Here's how the part is built. I have some questions about the finished solid (model axes, mm). Face numbers are marked on the shaded views. A direction names the side the tool comes from. Coordinates: 2 decimals unless noted, no trailing zeros. Write each loop counter-clockwise with the first axis right and the second up, starting at its lowest first coordinate (ties: lowest second). Pieces come first, ordered by that corner, then holes. Notation, with made-up numbers: (55.25, 88) -> (72.25, 88) arc R13 cw to (72.25, 108) -> close; hole circle Ø9 at (-19.5, -17). An arc over 180 degrees is marked (long way). Put each result on its own line as item: value.
```python
from build123d import *

# Parameters (mm, degrees)
BOSS_EXTRUDE1_DEPTH                             = 42
CUT_EXTRUDE1_DEPTH                              = 3
CUT_EXTRUDE2_DEPTH                              = 2
CSK_FOR_M3_FLAT_HEAD_MACHINE_SCREW1_D           = 3.4
CSK_FOR_M3_FLAT_HEAD_MACHINE_SCREW1_CSINK_D     = 6.3
CSK_FOR_M3_FLAT_HEAD_MACHINE_SCREW1_CSINK_ANGLE = 90
FILLET3_R                                       = 1
FILLET4_R                                       = 1
FILLET5_R                                       = 1
FILLET6_R                                       = 1
FILLET7_R                                       = 1
FILLET8_R                                       = 1


with BuildPart() as part:
    # Sketch1 → Boss-Extrude1 (new body)
    with BuildSketch(Plane.XY):
        Polygon((-124.373548005, 69.489611766), (-124.373548005, 24.489611766), (-109.373548005, 24.489611766), (-109.373548005, 28.489611766), (-120.373548005, 28.489611766), (-120.373548005, 69.489611766), align=None)
    extrude(amount=BOSS_EXTRUDE1_DEPTH)

    # Sketch2 → Cut-Extrude1 (cut)
    with BuildSketch(Plane(origin=(-120.373548005, 0, 0), x_dir=(0, 0, -1), z_dir=(1, 0, 0))):
        with BuildLine():
            Line((-42, 52.639611766), (-30, 52.639611766))
            ThreePointArc((-30, 52.639611766), (-26.35, 48.989611766), (-30, 45.339611766))
            Line((-30, 45.339611766), (-42, 45.339611766))
            Line((-42, 45.339611766), (-42, 52.639611766))
        make_face()
    cut_extrude1 = extrude(amount=-CUT_EXTRUDE1_DEPTH, mode=Mode.SUBTRACT)

    # Sketch4 → Cut-Extrude2 (cut, through all)
    with BuildSketch(Plane(origin=(-123.373548005, 0, 0), x_dir=(0, 0, -1), z_dir=(1, 0, 0))):
        with BuildLine():
            Line((-42, 51.189611766), (-42, 46.789611766))
            Line((-42, 46.789611766), (-30, 46.789611766))
            ThreePointArc((-30, 46.789611766), (-27.8, 48.989611766), (-30, 51.189611766))
            Line((-30, 51.189611766), (-42, 51.189611766))
        make_face()
    cut_extrude2 = extrude(amount=-CUT_EXTRUDE2_DEPTH, mode=Mode.SUBTRACT)

    # Mirror2: Cut-Extrude1, Cut-Extrude2 across plane
    add(cut_extrude1.mirror(Plane.XY.offset(21)), mode=Mode.SUBTRACT)
    add(cut_extrude2.mirror(Plane.XY.offset(21)), mode=Mode.SUBTRACT)

    # CSK for M3 Flat Head Machine Screw1 (through all)
    with Locations(Plane(origin=(0, 28.489611766, 0), x_dir=(1, 0, 0), z_dir=(0, 1, 0))):
        with Locations((-114.873548005, -32), (-114.873548005, -10)):
            CounterSinkHole(CSK_FOR_M3_FLAT_HEAD_MACHINE_SCREW1_D / 2, CSK_FOR_M3_FLAT_HEAD_MACHINE_SCREW1_CSINK_D / 2, counter_sink_angle=CSK_FOR_M3_FLAT_HEAD_MACHINE_SCREW1_CSINK_ANGLE)

    # Fillet3
    fillet3_edges = [part.edges().sort_by_distance(p)[0] for p in [
        (-120.373548005, 36.914611766, 42),
    ]]
    fillet(fillet3_edges, radius=FILLET3_R)

    # Fillet4
    fillet4_edges = [part.edges().sort_by_distance(p)[0] for p in [
        (-120.373548005, 61.064611766, 42),
    ]]
    fillet(fillet4_edges, radius=FILLET4_R)

    # Fillet5
    fillet5_edges = [part.edges().sort_by_distance(p)[0] for p in [
        (-120.666441224, 52.639611766, 41.707106781),
        (-122.373548005, 45.339611766, 42),
        (-122.373548005, 52.639611766, 42),
        (-120.373548005, 48.989611766, 26.35),
        (-120.373548005, 52.639611766, 35.5),
        (-120.373548005, 45.339611766, 35.5),
        (-120.666441224, 45.339611766, 41.707106781),
    ]]
    fillet(fillet5_edges, radius=FILLET5_R)

    # Fillet6
    fillet6_edges = [part.edges().sort_by_distance(p)[0] for p in [
        (-122.873548005, 69.489611766, 42),
        (-120.666441224, 69.489611766, 41.707106781),
        (-114.873548005, 28.489611766, 42),
        (-109.373548005, 28.489611766, 21),
        (-114.873548005, 28.489611766, 0),
        (-120.373548005, 36.914611766, 0),
        (-120.373548005, 48.989611766, 15.65),
        (-120.373548005, 45.339611766, 6),
        (-120.373548005, 52.639611766, 6),
        (-120.373548005, 61.064611766, 0),
        (-120.373548005, 69.489611766, 20.5),
    ]]
    fillet(fillet6_edges, radius=FILLET6_R)

    # Fillet7
    fillet7_edges = [part.edges().sort_by_distance(p)[0] for p in [
        (-123.873548005, 51.189611766, 42),
    ]]
    fillet(fillet7_edges, radius=FILLET7_R)

    # Fillet8
    fillet8_edges = [part.edges().sort_by_distance(p)[0] for p in [
        (-123.873548005, 46.789611766, 42),
        (-123.873548005, 51.189611766, 0),
        (-123.873548005, 46.789611766, 0),
    ]]
    fillet(fillet8_edges, radius=FILLET8_R)


solid = part.part
```
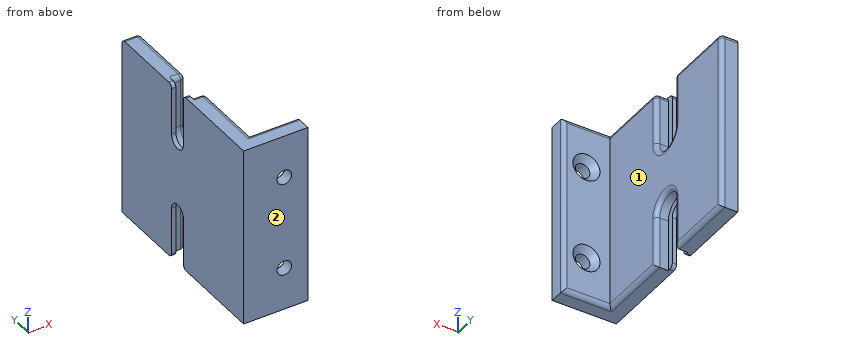
Item 1: Please list where these lines run through material, in increasing order: line 1 along Y through (x, z) = (-121.5, 3.5); line 2 along Y through (x, z) = (-118, 20.5); line 3 along X through (y, z) = (26, 10). Write a range as from..to.
Output:
line 1: y = 24.49..45.34, 52.64..69.49
line 2: y = 24.49..28.49
line 3: x = -124.37..-116.57, -113.17..-109.37
Item 2: Imagine slicing it at C-C on z = 10. Write out the boundary of the cut face in (x, y).
Output:
outline: (-124.37, 24.49) -> (-116.57, 24.49) -> (-116.57, 27.04) -> (-118.02, 28.49) -> (-120.37, 28.49) -> (-120.37, 44.34) arc R1 ccw to (-121.37, 45.34) -> (-123.37, 45.34) -> (-123.37, 46.79) -> (-124.37, 46.79) -> close; (-124.37, 51.19) -> (-123.37, 51.19) -> (-123.37, 52.64) -> (-121.37, 52.64) arc R1 ccw to (-120.37, 53.64) -> (-120.37, 68.49) arc R1 ccw to (-121.37, 69.49) -> (-124.37, 69.49) -> close; (-113.17, 24.49) -> (-109.37, 24.49) -> (-109.37, 27.49) arc R1 ccw to (-110.37, 28.49) -> (-111.72, 28.49) -> (-113.17, 27.04) -> close
Item 3: Imagine slicing it at A-A on z = 4. Write out the boundary of the cut face in (x, y).
Output:
outline: (-124.37, 24.49) -> (-109.37, 24.49) -> (-109.37, 27.49) arc R1 ccw to (-110.37, 28.49) -> (-120.37, 28.49) -> (-120.37, 44.34) arc R1 ccw to (-121.37, 45.34) -> (-123.37, 45.34) -> (-123.37, 46.79) -> (-124.37, 46.79) -> close; (-124.37, 51.19) -> (-123.37, 51.19) -> (-123.37, 52.64) -> (-121.37, 52.64) arc R1 ccw to (-120.37, 53.64) -> (-120.37, 68.49) arc R1 ccw to (-121.37, 69.49) -> (-124.37, 69.49) -> close
Item 4: Which directions (+Z, -Z, +X, -X, +Y, -Y) give clear straight access to the entire face, cutting with the end or side of a thin tool? Please do the marked faces 1 and 2.
Output:
face 1: +Z, -Z, +X, +Y
face 2: +Z, -Z, +X, -X, -Y
Item 5: Imagine slicing it at D-D on x = -115.75. State how many separate pieces and enclosed holes the cut face has, then the cut area to 3 significant figures.
Output:
separate pieces: 3
enclosed holes: 0
area: 140 mm²
Item 6: Imagine slicing it at B-B on y = 39.5. Write out the boundary of the cut face in (x, z), then the cut area to 3 significant figures.
Output:
outline: (-124.37, 0) -> (-121.37, 0) arc R1 ccw to (-120.37, 1) -> (-120.37, 41) arc R1 ccw to (-121.37, 42) -> (-124.37, 42) -> close
area: 168 mm²
Item 7: For P1, Ø3, axis at x = -113, z = 29.5, coming from the +Y side; P2, Ø10, axis at y = 47, z = 34.5, coming from the +X side; P3, Ø3, axis at x = -114.87, z = 32, coming from the +Y side; P4, Ø3, axis at x = -120, y = 49.5, coming from the -Z side, each with a flat end and sliding along its axis, tell me the tip position at first contact or that it passes through.
Output:
P1: stops at y = 28.49
P2: stops at x = -120.37
P3: passes through
P4: stops at z = 15.35
